from build123d import *

# Parameters (mm, degrees)
PAD_DEPTH = 10
FILLET_R  = 16


with BuildPart() as part:
    # Sketch → Pad (new body)
    with BuildSketch(Plane.XY):
        with BuildLine():
            Line((-278, -266.5), (-278, 266.5))
            Line((-278, 266.5), (278, 266.5))
            Line((278, 266.5), (278, -304))
            ThreePointArc((203, -304), (240.5, -341.5), (278, -304))
            Line((203, -266.5), (203, -304))
            Line((-278, -266.5), (203, -266.5))
        make_face()
        with BuildLine():
            Line((-216, 11.5), (-216, 199.5))
            Line((-216, 199.5), (216, 199.5))
            Line((216, 199.5), (216, 11.5))
            ThreePointArc((-216, 11.5), (0, -204.5), (216, 11.5))
        make_face(mode=Mode.SUBTRACT)
    extrude(amount=PAD_DEPTH)

    # Fillet
    fillet_edges = [part.edges().sort_by_distance(p)[0] for p in [
        (-216, 199.5, 5),
        (216, 199.5, 5),
    ]]
    fillet(fillet_edges, radius=FILLET_R)


solid = part.part
CAD build for the part. Positions are in the model's coordinates, mm. A direction names the side the tool comes from. Give positions to 0.01 mm unless a question says otherwise; leave off trailing zeros. Order: outer loops, then holes, each group sorted by start corner. A loop starts at its lowest first (then second) coordinate and runs counter-clockwise, first axis right, second up. Notation, with made-up numbers: (37.5, 56.25) - (57.5, 56.25) arc R27 cw to (57.5, 93.25) - close; hole circle Ø9 at (-20, 2). An arc over 180 degrees is marked (long way). Answer in a Markdown table with one row per item.
1. Flat gauge pin, fed straight in: pin 1 (5 mm diameter, centred on x = -75, z = 6, fed in from -Y). Where does the tip first touch, or does it go through?
Data:
| item | result |
|---|---|
| pin 1 | stops at y = -266.5 |
2. Pull direction X, two halves, no side cores. Call faces 1 (the flat face through (127, -168, 10)), 2 (the cylindrical face through (239.68, -341.49, 4.93)), 3 (the cylindrical face through (211.189, 194.937, 5.07)): pulls with the +X half, pulls with the -X half, needs draft (parallel to the pull), parting line crosses it, or undercut.
Data:
| item | result |
|---|---|
| face 1 | needs draft |
| face 2 | parting line crosses it |
| face 3 | undercut |
3. Saw through at A-A, the plane y = 41.5. Give the cut face in (x, z).
Data:
| item | result |
|---|---|
| outline | (-278, 0) - (-216, 0) - (-216, 10) - (-278, 10) - close; (216, 0) - (278, 0) - (278, 10) - (216, 10) - close |
4. Saw through at B-B, the plane z = 4.75. Give the cut face in (x, y).
Data:
| item | result |
|---|---|
| outline | (-278, -266.5) - (203, -266.5) - (203, -304) arc R37.5 ccw to (278, -304) - (278, 266.5) - (-278, 266.5) - close; hole (-216, 11.5) arc R216 ccw to (216, 11.5) - (216, 183.5) arc R16 ccw to (200, 199.5) - (-200, 199.5) arc R16 ccw to (-216, 183.5) - close |
5. Saw through at C-C, the plane x = 0. Give the cut face in (y, z).
Data:
| item | result |
|---|---|
| outline | (-266.5, 0) - (-204.5, 0) - (-204.5, 10) - (-266.5, 10) - close; (199.5, 0) - (266.5, 0) - (266.5, 10) - (199.5, 10) - close |
6. Tool access for faces 4 (the cylindrical face through (-4.75, -204.448, 4.93)), 5 (the flat face through (127, -168, 0)): list every direction of +Z, -Z, +X, -X, +Y, -Y with a clear straight run to the whole face (end or side of a thin tool).
Data:
| item | result |
|---|---|
| face 4 | +Z, -Z |
| face 5 | -Z, +X, -X, +Y, -Y |
7. Probe probe 1 along X at (y, z) = (148, 8.25); probe 2 along Y at (x, z) = (44, 6.5); probe 3 along Y at (x, z) = (156, 8.5). List the from-to ranges inside material, lowest first. Write a range as [from, to].
Data:
| item | result |
|---|---|
| probe 1 | x = [-278, -216], [216, 278] |
| probe 2 | y = [-266.5, -199.97], [199.5, 266.5] |
| probe 3 | y = [-266.5, -137.9], [199.5, 266.5] |
